The drawing under review shows one solid part. Ordinate dimensions are in mm from its lowest x, y, z. Coordinates: 2 decimals unless noted, no trailing zeros. Write each loop counter-clockwise with the first axis right and the second up, starting at its lowest first coordinate (ties: lowest second). Pieces come first, ordered by that corner, then holes.
Q1. Take a section at D-D (z = 9). Give the boundary of the cut face in (x, y).
Q2. Take a section at A-A (z = 28). Give the boundary of the cut face in (x, y).
Q3. Take a section at B-B (x = 28). Give the boundary of the cut face in (y, z).
Q4. For probe 1 along X at (y, z) = (3.25, 28); probe 2 along X at (y, z) = (2.15, 28); probe 3 along Y at (x, z) = (18.5, 6), list the stretches that pass through material, from the lowest coordinate up.
Q5. Insertion check: pin 1 (1.5 mm diameter, centred on y = 1.5, z = 45, fed in from -X); pin 2 (1 mm diameter, centred on x = 38, y = 1, fed in from +Z); pin 3 (2 mm diameter, centred on x = 11, y = 6, fed in from +Z). Each pin has a flat end and moves straight along its axis. Give the tip position at first contact, or say it passes through.
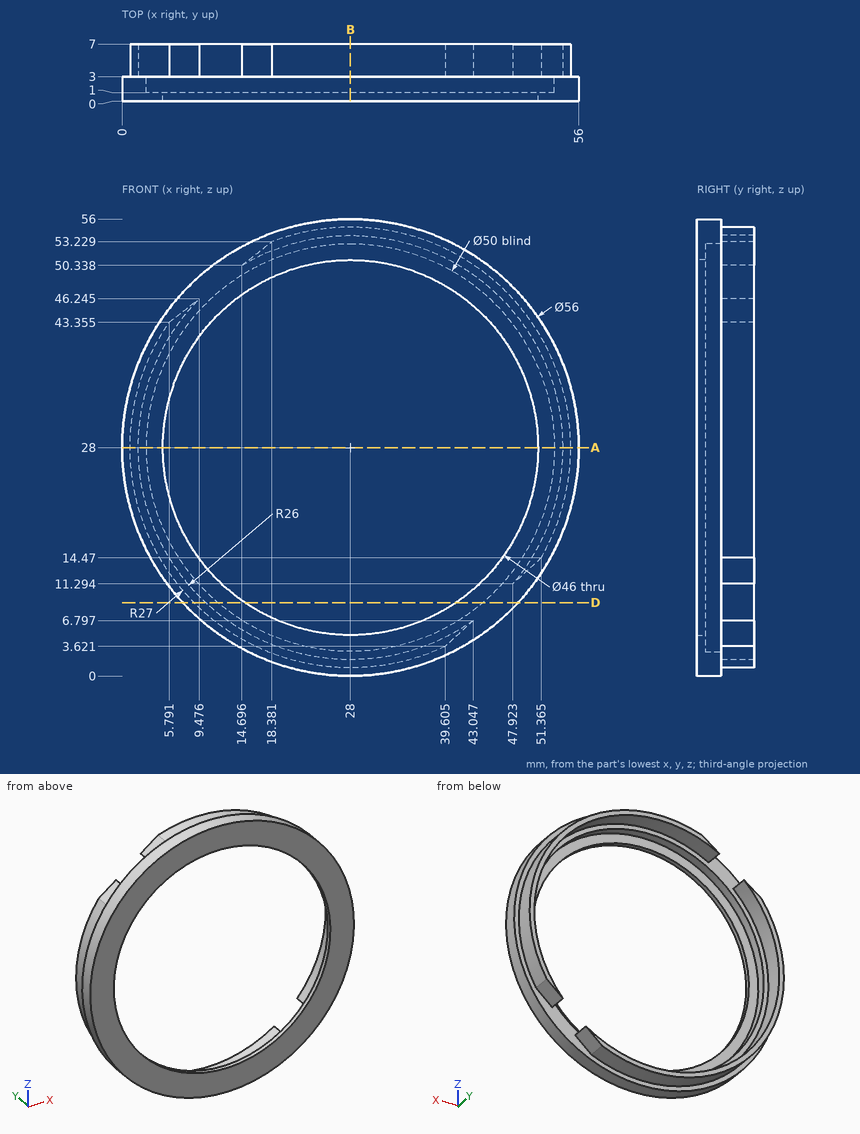
Response:
1. outline: (7.43, 0) - (15.04, 0) - (15.04, 1) - (11.75, 1) - (11.75, 3) - (10.25, 3) - (10.25, 7) - (8.82, 7) - (8.82, 3) - (7.43, 3) - close; (40.96, 0) - (48.57, 0) - (48.57, 3) - (44.25, 3) - (44.25, 1) - (40.96, 1) - close
2. outline: (0, 0) - (5, 0) - (5, 1) - (3, 1) - (3, 3) - (2, 3) - (2, 7) - (1, 7) - (1, 3) - (0, 3) - close; (51, 0) - (56, 0) - (56, 3) - (55, 3) - (55, 7) - (54, 7) - (54, 3) - (53, 3) - (53, 1) - (51, 1) - close
3. outline: (0, 0) - (3, 0) - (3, 1) - (7, 1) - (7, 2) - (3, 2) - (3, 3) - (1, 3) - (1, 5) - (0, 5) - close; (0, 51) - (1, 51) - (1, 53) - (3, 53) - (3, 54) - (7, 54) - (7, 55) - (3, 55) - (3, 56) - (0, 56) - close
4. probe 1: x = 1 to 2, 54 to 55
4. probe 2: x = 0 to 3, 53 to 56
4. probe 3: y = 0 to 1
5. pin 1: stops at x = 5.2
5. pin 2: stops at z = 54.34
5. pin 3: stops at z = 9.24
